Design review of the part built by this model. Coordinates are the model's own, in mm. Face numbers are marked on the shaded views. A direction names the side the tool comes from. Round coordinates to 2 decimals unless told otherwise and drop trailing zeros. Order: outer loops, then holes, each group sorted by start corner. A loop starts at its lowest first (then second) coordinate and runs counter-clockwise, first axis right, second up. Notation, with made-up numbers: M 41,67 L 54,67 A18 cw 54,91 Z; hole C 4,-33.5 d7. An arc over 180 degrees is marked long. Write each question's results on one line, items separated by ' | '. Start each with the question number.
Item 1: Take a section at C-C, the plane y = -7. Write out the cut boundary in (x, z), plus the area to 3 significant figures.
Item 2: Take a section at A-A, the plane z = 21.65. Write out the cut boundary in (x, y).
Item 3: Clearance check with flat-ended pins moving along their axes: pin 1 (1.5 mm diameter, centred on x = -1, z = 17, fed in from -Y); pin 2 (2 mm diameter, centred on x = -1.15, y = -7, fed in from +Z); pin 3 (2.5 mm diameter, centred on y = 2, z = 18, fed in from +X); pin 4 (1.8 mm diameter, centred on x = 0.35, z = 25.65, fed in from +Y). State where each tip first meets the part, or that it passes through.
Item 4: Take a section at B-B, the plane z = 3.5. Write out the cut boundary in (x, y).
Item 5: Take a section at D-D, the plane z = 9.25. Write out the cut boundary in (x, y), plus the area to 4 significant figures.
Item 6: Machinability: for the marked faces 1, 2 and 3, which of the approach directions +Z, -Z, +X, -X, +Y, -Y give a long, thin tool a straight path to every point of the face, cutting with its end or side? Answer none if there is none.
Item 7: Wall thickness on line 1 (Z direction, x = -4.25, y = -4.5); line 2 (X direction, y = -0.6, z = 18.15); line 3 (Y direction, x = -1.5, z = 3): over which ranges is each line inside the solid? List them lowest first. Write a range as [from, to].
```python
from build123d import *

# Parameters (mm, degrees)
BOSS_EXTRUDE1_DEPTH   = 30
SKETCH2_W             = 8
SKETCH2_H             = 4
BOSS_EXTRUDE2_DEPTH   = 10
SKETCH3_R             = 1
CUT_EXTRUDE1_DEPTH    = 10
M2_TAPPED_HOLE1_D     = 1.6
M2_TAPPED_HOLE1_DEPTH = 5.2
M2_TAPPED_HOLE1_TIP   = 0.480688495
M3_TAPPED_HOLE1_D     = 2.5
M3_TAPPED_HOLE1_DEPTH = 7.5
M3_TAPPED_HOLE1_TIP   = 0.751075774
CHAMFER1_SIZE         = 0.5


with BuildPart() as part:
    # Sketch1 → Boss-Extrude1 (new body)
    with BuildSketch(Plane.XY):
        Polygon((-5.152542373, 3), (-3.152542373, 3), (-3.152542373, 0), (-2.152542373, 0), (-2.152542373, 0.5), (2.847457627, 0.5), (2.847457627, -2), (-5.152542373, -2), align=None)
    extrude(amount=BOSS_EXTRUDE1_DEPTH)

    # Sketch2 → Boss-Extrude2 (add)
    with BuildSketch(Plane.XZ.offset(2)):
        with Locations((-1.152542373, 2)):
            Rectangle(SKETCH2_W, SKETCH2_H)
    extrude(amount=BOSS_EXTRUDE2_DEPTH)

    # Sketch3 → Cut-Extrude1 (cut)
    with BuildSketch(Plane(origin=(0, 0.5, 0), x_dir=(1, 0, 0), z_dir=(0, 1, 0))):
        with Locations((0.347457627, -18.15)):
            Circle(SKETCH3_R)
        with BuildLine():
            Line((-0.952542373, -14.65), (-0.952542373, -8.65))
            ThreePointArc((-0.952542373, -8.65), (0.347457627, -7.35), (1.647457627, -8.65))
            Line((1.647457627, -8.65), (1.647457627, -14.65))
            ThreePointArc((1.647457627, -14.65), (0.347457627, -15.95), (-0.952542373, -14.65))
        make_face()
    extrude(amount=-CUT_EXTRUDE1_DEPTH, mode=Mode.SUBTRACT)

    # M2 Tapped Hole1
    with Locations(Plane(origin=(0, 0.5, 0), x_dir=(1, 0, 0), z_dir=(0, 1, 0))):
        with Locations((0.347457627, -21.65), (0.347457627, -25.65)):
            Hole(M2_TAPPED_HOLE1_D / 2, depth=M2_TAPPED_HOLE1_DEPTH)
            with Locations((0, 0, -(M2_TAPPED_HOLE1_DEPTH + M2_TAPPED_HOLE1_TIP / 2))):  # 118° drill point
                Cone(0, M2_TAPPED_HOLE1_D / 2, M2_TAPPED_HOLE1_TIP, mode=Mode.SUBTRACT)

    # M3 Tapped Hole1
    with Locations(Plane.XY.offset(4)):
        with Locations((-1.152542373, -7)):
            Hole(M3_TAPPED_HOLE1_D / 2, depth=M3_TAPPED_HOLE1_DEPTH)
            with Locations((0, 0, -(M3_TAPPED_HOLE1_DEPTH + M3_TAPPED_HOLE1_TIP / 2))):  # 118° drill point
                Cone(0, M3_TAPPED_HOLE1_D / 2, M3_TAPPED_HOLE1_TIP, mode=Mode.SUBTRACT)

    # Chamfer1
    chamfer1_edges = [part.edges().sort_by_distance(p)[0] for p in [
        (2.847457627, -2, 17),
        (-5.152542373, -2, 17),
    ]]
    chamfer(chamfer1_edges, length=CHAMFER1_SIZE)


solid = part.part
```
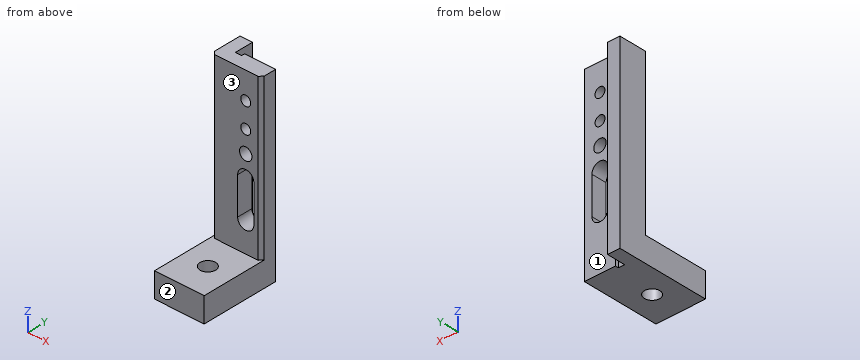
Results list:
1) outline: M -5.15,0 L -2.4,0 L -2.4,4 L -5.15,4 Z; M 0.1,0 L 2.85,0 L 2.85,4 L 0.1,4 Z | area: 22.0 mm²
2) outline: M -5.15,-1.5 L -4.65,-2 L -0.45,-2 L -0.45,0.5 L -2.15,0.5 L -2.15,0 L -3.15,0 L -3.15,3 L -5.15,3 Z; M 1.15,-2 L 2.35,-2 L 2.85,-1.5 L 2.85,0.5 L 1.15,0.5 Z
3) pin 1: y = -2 | pin 2: through | pin 3: x = -3.15 | pin 4: y = 0.5
4) outline: M -5.15,-12 L 2.85,-12 L 2.85,0.5 L -2.15,0.5 L -2.15,0 L -3.15,0 L -3.15,3 L -5.15,3 Z; hole C -1.15,-7 d2.5
5) outline: M -5.15,-1.5 L -4.65,-2 L -0.95,-2 L -0.95,0.5 L -2.15,0.5 L -2.15,0 L -3.15,0 L -3.15,3 L -5.15,3 Z; M 1.65,-2 L 2.35,-2 L 2.85,-1.5 L 2.85,0.5 L 1.65,0.5 Z | area: 17.75 mm²
6) face 1: +Z, -Z, +X, +Y | face 2: +Z, -Z, +X, -X, -Y | face 3: +Z, +X, -X, -Y
7) line 1: [0, 4] | line 2: [-5.15, -0.65], [1.35, 2.85] | line 3: [-12, -8.2], [-5.8, 0.5]
